Design review of the part shown in the three views and the two pictorial views. Dimensions are in mm from the part's minimum x, y and z. A direction names the side the tool comes from. Coordinates: 2 decimals unless noted, no trailing zeros. Write each loop counter-clockwise with the first axis right and the second up, starting at its lowest first coordinate (ties: lowest second). Pieces come first, ordered by that corner, then holes. Notation, with made-up numbers: (34.25, 33) -> (74.25, 33) arc R21 cw to (74.25, 40) -> close; hole circle Ø8 at (13.25, -26). An arc over 180 degrees is marked (long way). Answer in a Markdown table with one row per item. Add a question column.
Item 1: Clearance check with a flat-ended pin moving along its axis: P1, Ø5, axis at x = 23.5, y = 13.5, coming from the -Z side. State where the tip first meets the part, or that it passes through.
Item 2: To check wall thickness, follow line 1 (Y direction, x = 23.15, z = 1.3); line 2 (Y direction, x = 13, z = 1.9); line 3 (X direction, y = 13, z = 1.3). State the ranges of each line that lie inside material, in increasing order.
Item 3: Take a section at A-A, the plane y = 2.85. Write out the cut boundary in (x, z), and give its area (3 significant figures).
Item 4: Draft analysis for pull direction X (two halves, no side actions). For the marked faces 1, 2 and 3, state which applies: released by +X, released by -X, zero draft, split by the parting line, or undercut.
Item 5: For the marked faces 4 and 5, list the 3-axis set-ups (+Z, -Z, +X, -X, +Y, -Y) from which the entire face can be reached by the end or side of a thin tool; tool diameter is ignored.
Item 6: Take a section at C-C, the plane x = 23.15. Write out the cut boundary in (y, z).
Item 7: Take a section at B-B, the plane z = 2.95. Write out the cut boundary in (x, y).
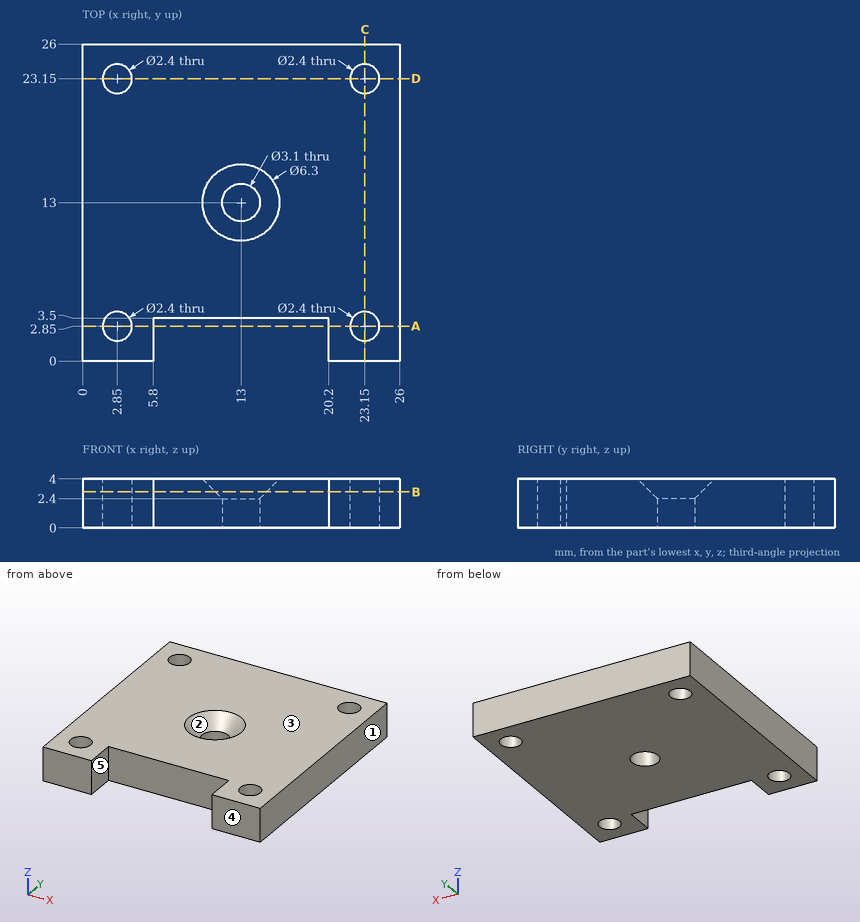
Answers:
| question | item | result |
|---|---|---|
| 1 | P1 | stops at z = 0 |
| 2 | line 1 | y = 0 to 1.65, 4.05 to 21.95, 24.35 to 26 |
| 2 | line 2 | y = 3.5 to 11.45, 14.55 to 26 |
| 2 | line 3 | x = 0 to 11.45, 14.55 to 26 |
| 3 | outline | (0, 0) -> (1.65, 0) -> (1.65, 4) -> (0, 4) -> close; (4.05, 0) -> (5.8, 0) -> (5.8, 4) -> (4.05, 4) -> close; (20.2, 0) -> (21.95, 0) -> (21.95, 4) -> (20.2, 4) -> close; (24.35, 0) -> (26, 0) -> (26, 4) -> (24.35, 4) -> close |
| 3 | area | 27.2 mm^2 |
| 4 | face 1 | released by +X |
| 4 | face 2 | undercut |
| 4 | face 3 | zero draft |
| 5 | face 4 | +Z, -Z, +X, -X, -Y |
| 5 | face 5 | +Z, -Z, -Y |
| 6 | outline | (0, 0) -> (1.65, 0) -> (1.65, 4) -> (0, 4) -> close; (4.05, 0) -> (21.95, 0) -> (21.95, 4) -> (4.05, 4) -> close; (24.35, 0) -> (26, 0) -> (26, 4) -> (24.35, 4) -> close |
| 7 | outline | (0, 0) -> (5.8, 0) -> (5.8, 3.5) -> (20.2, 3.5) -> (20.2, 0) -> (26, 0) -> (26, 26) -> (0, 26) -> close; hole circle Ø2.4 at (2.85, 2.85); hole circle Ø2.4 at (2.85, 23.15); hole circle Ø4.2 at (13, 13); hole circle Ø2.4 at (23.15, 2.85); hole circle Ø2.4 at (23.15, 23.15) |
